Design review of the part built by this model. Coordinates are the model's own, in mm. A direction names the side the tool comes from. Coordinates: 2 decimals unless noted, no trailing zeros. Write each loop counter-clockwise with the first axis right and the second up, starting at its lowest first coordinate (ties: lowest second). Pieces come first, ordered by that corner, then holes. Notation, with made-up numbers: (26.25, -23) - (36.25, -23) arc R6 ccw to (36.25, -13) - close; hole circle Ø1 at (-23.5, 59). An arc over 180 degrees is marked (long way). Answer as a JSON object with one key per item and string values.
```python
from build123d import *

# Parameters (mm, degrees)
F1_DEPTH = 15
F3_DEPTH = 70.001
F7_DEPTH = 6


with BuildPart() as f1:
    # F0 (on Front) → F1 (new body, symmetric)
    with BuildSketch(Plane.XZ):
        with BuildLine():
            Line((-35, 71), (-35, 0))
            Line((-35, 0), (35, 0))
            Line((35, 0), (35, 71))
            Line((35, 71), (15, 71))
            Line((15, 71), (15, 59))
            Line((15, 59), (18, 59))
            Line((18, 59), (21, 41))
            ThreePointArc((21, 41), (0, 20), (-21, 41))
            Line((-21, 41), (-18, 59))
            Line((-18, 59), (-15, 59))
            Line((-15, 59), (-15, 71))
            Line((-15, 71), (-35, 71))
        make_face()
    extrude(amount=F1_DEPTH, both=True)

    # F2 (on face) → F3 (cut, through all)
    with BuildSketch(Plane(origin=(-35, 0, 0), x_dir=(0, -1, 0), z_dir=(-1, 0, 0))):
        Polygon((-10, 71), (-15, 71), (-15, 0), align=None)
        Polygon((10, 71), (15, 0), (15, 71), align=None)
    extrude(amount=-F3_DEPTH, mode=Mode.SUBTRACT)

    # F4 (on Front) → F5 (revolve)
    with BuildSketch(Plane.XZ):
        Polygon((10, 0), (0, 0), (0, -35), (10, -35), (10, -31), (7, -31), (7, -26), (10, -26), align=None)
    revolve(axis=Axis((0, 0, -17.5), (0, 0, -1)))

    # F6 (on face) → F7 (cut)
    with BuildSketch(Plane(origin=(0, 0, -35), x_dir=(1, 0, 0), z_dir=(0, 0, -1))):
        with BuildLine():
            Line((17, 0), (7, 0))
            ThreePointArc((7, 0), (0, -7), (-7, 0))
            Line((-7, 0), (-17, 0))
            Line((-17, 0), (-17, -25.996203))
            Line((-17, -25.996203), (17, -25.996203))
            Line((17, -25.996203), (17, 0))
        make_face()
    extrude(amount=-F7_DEPTH, mode=Mode.SUBTRACT)


solid = f1.part
```
(1) Take a section at C-C, the plane x = -23.5. Write out the cut boundary in (y, z).
Solved:
{"outline": "(-15, 0) - (15, 0) - (10, 71) - (-10, 71) - close"}
(2) The part is to be moulded in two halves that separate along X. For faces 1 (the face through (3.23, 6.21, -29.44)), 2 (the face through (35, 0, 35)), 3 (the face through (0, 0, 20)), say which applies: pulls with the +X half, pulls with the -X half, needs draft (parallel to the pull), parting line crosses it, or undercut.
Solved:
{"face 1": "parting line crosses it", "face 2": "pulls with the +X half", "face 3": "undercut"}
(3) Take a section at B-B, the plane z = -17. Write out the cut boundary in (x, y), and give its area (3 significant figures).
Solved:
{"outline": "circle Ø20 at (0, 0)", "area": "314 mm^2"}
(4) For pin 1 (1.5 mm diameter, centred on x = 8.5, z = -34, fed in from +Y); pin 2 (1 mm diameter, centred on x = 14, y = 6.5, fed in from +Z); pin 3 (12 mm diameter, centred on x = 22, z = 57.5, fed in from +Y), all flat-tipped, find the tip position at first contact; note any pin that passes through.
Solved:
{"pin 1": "stops at y = 0", "pin 2": "stops at z = 25.81", "pin 3": "stops at y = 11.37"}
(5) To check wall thickness, follow line 1 (Z direction, x = -29, y = 3); line 2 (X direction, y = -3.25, z = 22); line 3 (Z direction, x = -7, y = -0.75). State the ranges of each line that lie inside material, in increasing order. Write a range as from..to.
Solved:
{"line 1": "z = 0..71", "line 2": "x = -35..-8.94, 8.94..35", "line 3": "z = -35..-31, -26..21.2"}
(6) Take a section at A-A, the plane x = 0. Write out the cut boundary in (y, z), and give its area (3 significant figures).
Solved:
{"outline": "(-15, 0) - (-10, 0) - (-10, -26) - (-7, -26) - (-7, -31) - (-10, -31) - (-10, -35) - (7, -35) - (7, -26) - (10, -26) - (10, 0) - (15, 0) - (13.59, 20) - (-13.59, 20) - close", "area": "1,230 mm^2"}
(7) Tool access review of faces 4 (the face through (19.48, -0.17, 50.13)), 5 (the face through (0, -10, -33)), 6 (the face through (-2.17, 9.76, -12.82)): name each direction out of +Z, -Z, +X, -X, +Y, -Y from which nothing blocks a thin tool from reaching the whole face with its end or side.
Solved:
{"face 4": "+Y, -Y", "face 5": "-Z, -Y", "face 6": "-Z"}
(8) Take a section at D-D, the plane z = 4. Write out the cut boundary in (x, y).
Solved:
{"outline": "(-35, -14.72) - (35, -14.72) - (35, 14.72) - (-35, 14.72) - close"}
